```python
from build123d import *

# Parameters (mm, degrees)
SKETCH1_W      = 228.04397219
SKETCH1_H      = 10.103213958
EXTRUDE1_DEPTH = 10
EXTRUDE2_DEPTH = 10
EXTRUDE3_DEPTH = 10


with BuildPart() as part:
    # Sketch1 → Extrude1 (new body)
    with BuildSketch(Plane.XY):
        with Locations((0, 48.080473567)):
            Rectangle(SKETCH1_W, SKETCH1_H)
    extrude(amount=EXTRUDE1_DEPTH)



with BuildPart() as body_2:
    # Sketch1<3> → Extrude2 (new body)
    with BuildSketch(Plane.XY):
        Polygon((40.232441296, -51.869178801), (40.232441296, -41.765964843), (30.129227338, -41.765964843), (-29.768398268, -41.765964843), (-39.871612226, -41.765964843), (-39.871612226, -51.869178801), align=None)
    extrude(amount=EXTRUDE2_DEPTH)


with BuildPart() as part_1:
    add(part.part)

    add(body_2.part)  # Extrude3 merges body 2
    # Sketch1<4> → Extrude3 (add)
    with BuildSketch(Plane.XY):
        Polygon((40.232441296, -41.765964843), (73.609130264, 43.028866588), (63.686330841, 43.028866588), (30.129227338, -41.765964843), align=None)
        Polygon((-29.768398268, -41.765964843), (-63.505916306, 43.028866588), (-73.609130264, 43.028866588), (-39.871612226, -41.765964843), align=None)
    extrude(amount=EXTRUDE3_DEPTH)


solid = part_1.part
```
Geometry check sheet. Reference: the model listing, model coordinates, mm. A direction names the side the tool comes from. Coordinates: 2 decimals unless noted, no trailing zeros. Write each loop counter-clockwise with the first axis right and the second up, starting at its lowest first coordinate (ties: lowest second). Pieces come first, ordered by that corner, then holes. Notation, with made-up numbers: M 3.5,6.25 L 24.5,6.25 A7 cw 24.5,19.25 Z; hole C 65,27 d10. An arc over 180 degrees is marked long. Use one line per item in the form item = value. Start each with the question number.
1) Section check A-A on x = -6. Enter the section's corners in (y, z), and give its area (3 significant figures).
2) Go/stop test with flat-tipped pins: pin 1 Ø5 at (x, z) = (91, 6) entering from -Y; pin 2 Ø3 at (y, z) = (-32, 1.5) entering from -X; pin 3 Ø5 at (y, z) = (-49, 2.5) entering from +X. Record where each tip stops, or that it passes through.
3) Section check C-C on y = 21. Enter the section's corners in (x, z).
4) Section check B-B on z = 2.5. Enter the section's corners in (x, y), and give its area (3 significant figures).
5) Set-up check for faces 1 (the flat face through (0, -51.869, 5)), 2 (the flat face through (1, -41.766, 5)), 3 (the flat face through (-94, 43.029, 5)), 4 (the flat face through (40.232, -47, 5)): record each of +Z, -Z, +X, -X, +Y, -Y from which the full face is reachable in a straight line by a thin tool's end or side.
6) Thickness scan on probe 1 along Y at (x, z) = (8.5, 3); probe 2 along Y at (x, z) = (102.5, 6); probe 3 along X at (y, z) = (14, 3.25). Record the ranges inside material, lowest first. Write a range as from..to.
7) Section check D-D on x = -83. Enter the section's corners in (y, z).
8) Release check for a two-part mould opening along X. For faces 5 (the flat face through (94, 43.029, 5)), 6 (the flat face through (-39.872, -47, 5)), 7 (the flat face through (56.69, 0.04, 4.93)), 8 (the flat face through (-46.4, 0.04, 4.93)) record: pulls with the +X half, pulls with the -X half, needs draft (parallel to the pull), parting line crosses it, or undercut.
Responses:
q1.outline = M -51.87,0 L -41.77,0 L -41.77,10 L -51.87,10 Z; M 43.03,0 L 53.13,0 L 53.13,10 L 43.03,10 Z
q1.area = 202 mm2
q2.pin_1 = 43.03
q2.pin_2 = -44.35
q2.pin_3 = 40.23
q3.outline = M -64.84,0 L -54.74,0 L -54.74,10 L -64.84,10 Z; M 54.97,0 L 64.94,0 L 64.94,10 L 54.97,10 Z
q4.outline = M -114.02,43.03 L -73.61,43.03 L -39.87,-41.77 L -39.87,-51.87 L 40.23,-51.87 L 40.23,-41.77 L 73.61,43.03 L 114.02,43.03 L 114.02,53.13 L -114.02,53.13 Z; hole M -63.51,43.03 L -29.77,-41.77 L 30.13,-41.77 L 63.69,43.03 Z
q4.area = 4,820 mm2
q5.face_1 = +Z, -Z, +X, -X, -Y
q5.face_2 = +Z, -Z
q5.face_3 = +Z, -Z, -X, -Y
q5.face_4 = +Z, -Z, +X, -Y
q6.probe_1 = -51.87..-41.77, 43.03..53.13
q6.probe_2 = 43.03..53.13
q6.probe_3 = -62.06..-51.96, 52.2..62.18
q7.outline = M 43.03,0 L 53.13,0 L 53.13,10 L 43.03,10 Z
q8.face_5 = needs draft
q8.face_6 = pulls with the -X half
q8.face_7 = pulls with the +X half
q8.face_8 = undercut
